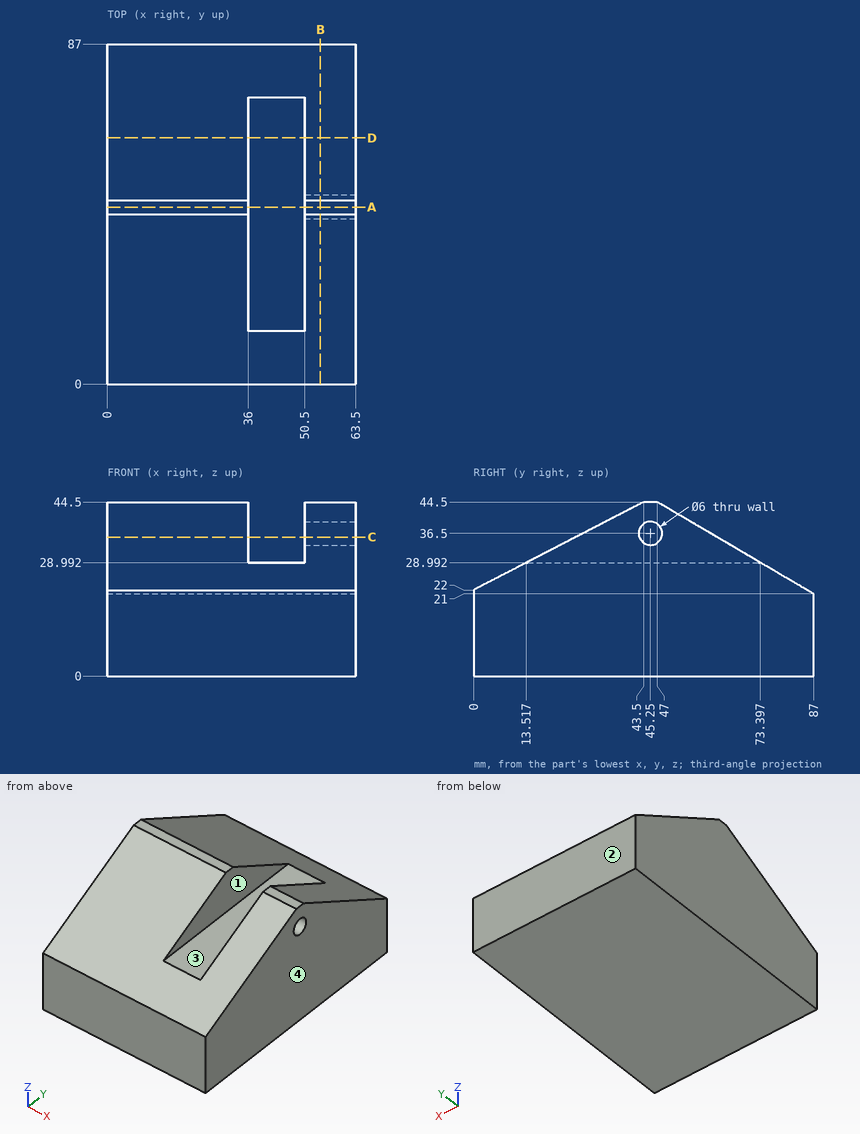
Geometry: see drawing. Coordinates: mm, zero at the bounding-box minimum. Round coordinates to 2 decimals unless told otherwise and drop trailing zeros. Order: outer loops, then holes, each group sorted by start corner. A loop starts at its lowest first (then second) coordinate and runs counter-clockwise, first axis right, second up. Notation, with made-up numbers: (9, 21) -> (61, 21) arc R7 ccw to (61, 33) -> close; hole circle Ø4 at (-31.5, -23). An arc over 180 degrees is marked (long way). Write each question's results on one line, items separated by ' | '.
Q1. Pull-direction query (X, two-part tool) for the marked faces 1, 2, 3 and 4; classes: released by +X, released by -X, zero draft, split by the parting line, or undercut.
Response values:
face 1: undercut | face 2: zero draft | face 3: undercut | face 4: released by +X
Q2. Pin query (flat end, axial travel): pin 1 Ø11.5 at (x, y) = (45, 38) entering from +Z; pin 2 Ø1.5 at (x, y) = (12.5, 39.5) entering from +Z; pin 3 Ø4 at (x, y) = (26.5, 52.5) entering from +Z. Return the tip coordinate at first contact, or that it passes through.
Response values:
pin 1: z = 42.52 | pin 2: z = 42.82 | pin 3: z = 42.44
Q3. Section query A-A (y = 45.25). Output: boundary loops of the cut face in (x, z).
Response values:
outline: (0, 0) -> (63.5, 0) -> (63.5, 33.5) -> (50.5, 33.5) -> (50.5, 28.99) -> (36, 28.99) -> (36, 44.5) -> (0, 44.5) -> close; (50.5, 39.5) -> (63.5, 39.5) -> (63.5, 44.5) -> (50.5, 44.5) -> close
Q4. Ray query, line 1 along Z through (x, y) = (56, 45.25); line 2 along X through (y, z) = (44.5, 41); line 3 along Z through (x, y) = (8.5, 74). Return the intervals inside material, ascending.
Response values:
line 1: 0 to 33.5, 39.5 to 44.5 | line 2: 0 to 36, 50.5 to 63.5 | line 3: 0 to 28.64
Q5. Section query B-B (x = 54.5). Output: boundary loops of the cut face in (y, z).
Response values:
outline: (0, 0) -> (87, 0) -> (87, 21) -> (47, 44.5) -> (43.5, 44.5) -> (0, 22) -> close; hole circle Ø6 at (45.25, 36.5)
Q6. Section query D-D (y = 63). Output: boundary loops of the cut face in (x, z).
Response values:
outline: (0, 0) -> (63.5, 0) -> (63.5, 35.1) -> (50.5, 35.1) -> (50.5, 28.99) -> (36, 28.99) -> (36, 35.1) -> (0, 35.1) -> close
Q7. Section query C-C (z = 35.5). Output: boundary loops of the cut face in (x, y), and give its area (3 significant figures).
Response values:
outline: (0, 26.1) -> (36, 26.1) -> (36, 62.32) -> (0, 62.32) -> close; (50.5, 26.1) -> (63.5, 26.1) -> (63.5, 42.42) -> (50.5, 42.42) -> close; (50.5, 48.08) -> (63.5, 48.08) -> (63.5, 62.32) -> (50.5, 62.32) -> close | area: 1,700 mm²
